The listing builds one solid part. Answer for the finished solid, in the listing's coordinates (mm). A direction names the side the tool comes from. Give positions to 0.01 mm unless a question says otherwise; leave off trailing zeros. Loops run counter-clockwise (first coordinate to the right, second up) from the corner with the lowest first, then second, coordinate; pieces in that order, holes last. Notation, with made-up numbers: (88.25, 67) - (119.25, 67) arc R25 cw to (119.25, 97) - close; hole circle Ø6 at (-7.75, 68.25). An arc over 180 degrees is marked (long way). Write each question's results on one line, items separated by ' | '.
Autodesk Fusion 360 part; units mm, degrees
sketch "Sketch1" plane through (0, 0, 0) normal (0, 0, 1) x (1, 0, 0)
  line L0 (10.1, -17.15) -> (-10.1, -17.15)
  line L1 (-10.1, -17.15) -> (-10.1, 17.15)
  line L2 (-10.1, 17.15) -> (10.1, 17.15)
  line L3 (10.1, 17.15) -> (10.1, -17.15)
  line L4 (10.1, -17.15) -> (-10.1, 17.15) construction
  line L5 (-10.1, -17.15) -> (10.1, 17.15) construction
  line L6 (11.7, 18.75) -> (-11.7, 18.75)
  line L7 (-11.7, 18.75) -> (-11.7, -18.75)
  line L8 (-11.7, -18.75) -> (11.7, -18.75)
  line L9 (11.7, -18.75) -> (11.7, 18.75)
  line L10 (11.7, 18.75) -> (-11.7, -18.75) construction
  line L11 (-11.7, 18.75) -> (11.7, -18.75) construction
  dimension "d1" = 20.2
  dimension "d2" = 34.3
  dimension "d4" = 1.6
  dimension "d5" = 1.6
extrude "Extrude1" add sketch "Sketch1" along normal blind 8
sketch "Sketch2" plane through (0, 0, 0) normal (0, 0, -1) x (1, 0, 0)
  line L0 (10.1, -17.15) -> (-10.1, -17.15)
  line L1 (-10.1, -17.15) -> (-10.1, 17.15)
  line L2 (-10.1, 17.15) -> (10.1, 17.15)
  line L3 (10.1, 17.15) -> (10.1, -17.15)
  line L4 (11.7, -18.75) -> (11.7, 18.75)
  line L5 (11.7, 18.75) -> (-11.7, 18.75)
  line L6 (-11.7, 18.75) -> (-11.7, -18.75)
  line L7 (-11.7, -18.75) -> (11.7, -18.75)
  line L8 (-11.7, 18.75) -> (11.7, 18.75)
  line L9 (11.7, 18.75) -> (11.7, -18.75)
  line L10 (11.7, -18.75) -> (-11.7, -18.75)
  line L11 (-11.7, -18.75) -> (-11.7, 18.75)
extrude "Extrude2" add sketch "Sketch2" along normal blind 1.4 contours L0 L1 L2 L3 | L4 L5 L6 L7 L8 L9 L10 L11
sketch "Sketch3" plane through (0, -18.75, 0) normal (0, -1, 0) x (1, 0, 0)
  line L0 (11.7, -1.4) -> (11.7, 8)
  line L1 (11.7, 8) -> (-11.7, 8)
  line L2 (-11.7, 8) -> (-11.7, -1.4)
  line L3 (-11.7, -1.4) -> (11.7, -1.4)
  line L4 (-5.52, 8) -> (4.08, 8)
  line L5 (4.08, 8) -> (4.08, 5.6)
  line L6 (4.08, 5.6) -> (-5.52, 5.6)
  line L7 (-5.52, 5.6) -> (-5.52, 8)
  dimension "d10" = 7
  dimension "d11" = 6.18
  dimension "d14" = 9.6
extrude "Extrude3" cut sketch "Sketch3" against normal up to surface (1.6 mm away) contours L1 L4 L5 L6 L7
fillet "Fillet1" radius 1.3 2 edges at (-5.52, -17.95, 5.6) (4.08, -17.95, 5.6)
sketch "Sketch4" plane through (-11.7, 0, 0) normal (-1, 0, 0) x (0, -1, 0)
  line L0 (18.75, -1.4) -> (18.75, 8)
  line L1 (18.75, 8) -> (-18.75, 8)
  line L2 (-18.75, 8) -> (-18.75, -1.4)
  line L3 (-18.75, -1.4) -> (18.75, -1.4)
  line L4 (10.55, 7.65) -> (15.55, 7.65)
  line L5 (15.55, 7.65) -> (15.55, 6.45)
  line L6 (15.55, 6.45) -> (10.55, 6.45)
  line L7 (10.55, 6.45) -> (10.55, 7.65)
  dimension "d17" = 3.2
  dimension "d18" = 5
  dimension "d19" = 1.2
  dimension "d22" = 0.35
extrude "Extrude4" cut sketch "Sketch4" against normal up to surface (1.6 mm away) contours L4 L5 L6 L7
fillet "Fillet2" radius 0.15 4 edges at (-11.7, -13.05, 6.45) (-11.7, -10.55, 7.05) (-11.7, -13.05, 7.65) (-11.7, -15.55, 7.05)
sketch "Sketch5" plane through (0, 0, 8) normal (0, 0, 1) x (-1, 0, 0)
  line L0 (-4.08, 17.15) -> (-4.08, 18.75)
  line L1 (-4.08, 18.75) -> (-11.7, 18.75)
  line L2 (-11.7, 18.75) -> (-11.7, -18.75)
  line L3 (-11.7, -18.75) -> (11.7, -18.75)
  line L4 (11.7, -18.75) -> (11.7, 18.75)
  line L5 (11.7, 18.75) -> (5.52, 18.75)
  line L6 (5.52, 18.75) -> (5.52, 17.15)
  line L7 (5.52, 17.15) -> (10.1, 17.15)
  line L8 (10.1, 17.15) -> (10.1, -17.15)
  line L9 (10.1, -17.15) -> (-10.1, -17.15)
  line L10 (-10.1, -17.15) -> (-10.1, 17.15)
  line L11 (-10.1, 17.15) -> (-4.08, 17.15)
  line L12 (10.9, -17.95) -> (-10.9, -17.95)
  line L13 (-10.9, -17.95) -> (-10.9, 17.95)
  line L14 (-10.9, 17.95) -> (10.9, 17.95)
  line L15 (10.9, 17.95) -> (10.9, -17.95)
  dimension "d26" = 0.8
  dimension "d27" = 0.8
  dimension "d28" = 0.8
  dimension "d29" = 0.8
extrude "Extrude5" add sketch "Sketch5" along normal blind 1.5 contours L0 L6 L7 L8 L9 L10 L11 L12 L13 L14 L15
sketch "Sketch7" plane through (10.9, 0, 0) normal (1, 0, 0) x (0, 1, 0)
  line L0 (-17.95, 8) -> (17.95, 8)
  line L1 (17.95, 8) -> (17.95, 9.5)
  line L2 (17.95, 9.5) -> (-17.95, 9.5)
  line L3 (-17.95, 9.5) -> (-17.95, 8)
  line L4 (-17.95, 9.5) -> (17.95, 8) construction
  line L5 (17.95, 9.5) -> (-17.95, 8) construction
  line L6 (0, 8.75) -> (-14.5, 8.75) construction
  line L7 (7.5, 8.45) -> (-7.5, 8.45)
  line L8 (-7.5, 8.45) -> (-7.5, 9.05)
  line L9 (-7.5, 9.05) -> (7.5, 9.05)
  line L10 (7.5, 9.05) -> (7.5, 8.45)
  line L11 (7.5, 8.45) -> (-7.5, 9.05) construction
  line L12 (-7.5, 8.45) -> (7.5, 9.05) construction
  point P0 (0, 8.75)
  dimension "d32" = 15
  dimension "d33" = 0.6
ref_plane "WorkPlane1" through (0, 0, 8.75) normal (1, 0, 0) x (0, 1, 0)
extrude "Extrude6" cut sketch "Sketch7" against normal blind 0.45 contours L7 L8 L9 L10
fillet "Fillet5" radius 0.2 4 edges at (10.675, -7.5, 8.45) (10.675, -7.5, 9.05) (10.675, 7.5, 8.45) (10.675, 7.5, 9.05)
fillet "Fillet6" radius 0.2 8 edges at (10.9, -7.4414, 8.5086) (10.9, 0, 8.45) (10.9, 7.4414, 8.5086) (10.9, 7.5, 8.75) (10.9, 7.4414, 8.9914) (10.9, 0, 9.05) (10.9, -7.4414, 8.9914) (10.9, -7.5, 8.75)
mirror "Mirror2" about plane through (0, 0, 8.75) normal (1, 0, 0) of "Extrude6"
fillet "Fillet7" radius 0.2 4 edges at (-10.675, 7.5, 8.45) (-10.675, 7.5, 9.05) (-10.675, -7.5, 8.45) (-10.675, -7.5, 9.05)
fillet "Fillet8" radius 0.2 8 edges at (-10.9, -7.4414, 8.9914) (-10.9, -7.5, 8.75) (-10.9, -7.4414, 8.5086) (-10.9, 0, 8.45) (-10.9, 7.4414, 8.5086) (-10.9, 7.5, 8.75) (-10.9, 7.4414, 8.9914) (-10.9, 0, 9.05)
fillet "Fillet9" radius 0.5 8 edges at (-11.7, 18.75, 3.3) (-11.7, -18.75, 3.3) (-11.7, 0, -1.4) (0, -18.75, -1.4) (11.7, -18.75, 3.3) (11.7, 0, -1.4) (11.7, 18.75, 3.3) (0, 18.75, -1.4)
sketch "Sketch8" plane through (0, 17.15, 0) normal (0, -1, 0) x (1, 0, 0)
  line L0 (-10.1, 0) -> (10.1, 0)
  line L1 (10.1, 0) -> (10.1, 9.5)
  line L2 (10.1, 9.5) -> (-10.1, 9.5)
  line L3 (-10.1, 9.5) -> (-10.1, 0)
  line L4 (4, 7.5) -> (5.5, 7.5)
  line L5 (5.5, 7.5) -> (5.5, 6.5)
  line L6 (5.5, 6.5) -> (4, 6.5)
  line L7 (4, 6.5) -> (4, 7.5)
  dimension "d55" = 4.6
  dimension "d56" = 1
  dimension "d57" = 1.5
  dimension "d58" = 2
extrude "Extrude7" cut sketch "Sketch8" against normal up to surface (1.6 mm away) contours L4 L5 L6 L7
fillet "Fillet10" radius 0.3 4 edges at (5.5, 17.95, 6.5) (5.5, 17.95, 7.5) (4, 17.95, 7.5) (4, 17.95, 6.5)
equation "case_thickness = 1.6 mm"
equation "d4 = case_thickness"
equation "d5 = case_thickness"
equation "d8 = case_thickness - 0.2 mm"
equation "d11 = 4.58 mm + case_thickness"
equation "lock_rim = 0.8 mm"
equation "d26 = lock_rim"
equation "d27 = lock_rim"
equation "d28 = lock_rim"
equation "d29 = lock_rim"
equation "d43 = clip_roundness"
equation "d45 = clip_roundness"
equation "clip_roundness = 0.2 mm"
equation "d50 = clip_roundness"
equation "d52 = clip_roundness"
Item 1: A cutting plane is placed at B-B, the plane x = -3.75. Determine the outline of the cut face in (y, z), plus the area to 3 significant figures.
Values found:
outline: (-18.75, -0.9) arc R0.5 ccw to (-18.25, -1.4) - (18.25, -1.4) arc R0.5 ccw to (18.75, -0.9) - (18.75, 8) - (17.95, 8) - (17.95, 9.5) - (17.15, 9.5) - (17.15, 0) - (-17.15, 0) - (-17.15, 5.6) - (-18.75, 5.6) - close | area: 75.4 mm²
Item 2: A cutting plane is placed at A-A, the plane z = 1.5. Determine the outline of the cut face in (x, y), plus the area to 3 significant figures.
Values found:
outline: (-11.7, -18.25) arc R0.5 ccw to (-11.2, -18.75) - (11.2, -18.75) arc R0.5 ccw to (11.7, -18.25) - (11.7, 18.25) arc R0.5 ccw to (11.2, 18.75) - (-11.2, 18.75) arc R0.5 ccw to (-11.7, 18.25) - close; hole (-10.1, -17.15) - (10.1, -17.15) - (10.1, 17.15) - (-10.1, 17.15) - close | area: 184 mm²
Item 3: A cutting plane is placed at C-C, the plane y = 4.5. Determine the outline of the cut face in (x, z).
Values found:
outline: (-11.7, -0.9) arc R0.5 ccw to (-11.2, -1.4) - (11.2, -1.4) arc R0.5 ccw to (11.7, -0.9) - (11.7, 8) - (10.9, 8) - (10.9, 8.25) arc R0.2 ccw to (10.7, 8.45) - (10.45, 8.45) - (10.45, 9.05) - (10.7, 9.05) arc R0.2 ccw to (10.9, 9.25) - (10.9, 9.5) - (10.1, 9.5) - (10.1, 0) - (-10.1, 0) - (-10.1, 9.5) - (-10.9, 9.5) - (-10.9, 9.25) arc R0.2 ccw to (-10.7, 9.05) - (-10.45, 9.05) - (-10.45, 8.45) - (-10.7, 8.45) arc R0.2 ccw to (-10.9, 8.25) - (-10.9, 8) - (-11.7, 8) - close
Item 4: For a pull along Z with two mould halves and no side action, classify faces 1 (the face through (-11, -15.55, 7)), 2 (the face through (-11.7, 0, 3)), 3 (the face through (3.71, -17.94, 5.99)) as released by +Z, released by -Z, zero draft, split by the parting line, or undercut.
Values found:
face 1: undercut | face 2: zero draft | face 3: released by +Z
Item 5: Flat-ended cylindrical pins translate along their axes: P1, Ø8, axis at x = -1, y = 3, coming from the +Z side; P2, Ø0.5, axis at y = -3.5, z = 9, coming from the -X side; P3, Ø0.5, axis at x = -1.5, y = -18.5, coming from the +Z side. Find the tip coordinate at first contact, or state that the pin passes through.
Values found:
P1: stops at z = 0 | P2: stops at x = -10.9 | P3: stops at z = 5.6
Item 6: A cutting plane is placed at D-D, the plane y = 9. Determine the outline of the cut face in (x, z), plus the area to 3 significant figures.
Values found:
outline: (-11.7, -0.9) arc R0.5 ccw to (-11.2, -1.4) - (11.2, -1.4) arc R0.5 ccw to (11.7, -0.9) - (11.7, 8) - (10.9, 8) - (10.9, 9.5) - (10.1, 9.5) - (10.1, 0) - (-10.1, 0) - (-10.1, 9.5) - (-10.9, 9.5) - (-10.9, 8) - (-11.7, 8) - close | area: 60.7 mm²
Item 7: Find the intervals of material crossed by line 1 along X through (y, z) = (8.5, 1); line 2 along Y through (x, z) = (-2.25, 4); line 3 along X through (y, z) = (17, 9.25), in increasing order. Write a range as [from, to].
Values found:
line 1: x = [-11.7, -10.1], [10.1, 11.7] | line 2: y = [-18.75, -17.15], [17.15, 18.75] | line 3: x = [-10.9, -10.1], [10.1, 10.9]
Item 8: For faces 4 (the face through (-11, -13, 6.45)), 5 (the face through (-11.3, 1.5, 8)), 6 (the face through (-5.52, -17.8, 7.9)), 7 (the face through (5, 18, 7.5)), 8 (the face through (11.7, 0, 3)), determine the directions among +Z, -Z, +X, -X, +Y, -Y from which every point of the face is accessible in a straight line to the end or side of a thin tool.
Values found:
face 4: -X | face 5: +Z | face 6: +Z, -Y | face 7: +Y | face 8: +Z, -Z, +X, +Y, -Y
